```python
from build123d import *

# Parameters (mm, degrees)
SKETCH1_R                 = 1.143
BOSS_EXTRUDE1_DEPTH       = 3.9624
SKETCH2_W                 = 6.35
SKETCH2_H                 = 4.7752
BOSS_EXTRUDE2_DEPTH       = 7.2136
BOSS_EXTRUDE3_DEPTH       = 0.127
BOSS_EXTRUDE3_DEPTH_BACK  = 0.127
SKETCH3_R                 = 0.5588
BOSS_EXTRUDE4_DEPTH       = 0.127
BOSS_EXTRUDE4_DEPTH_BACK  = 0.127
SKETCH4_R                 = 0.5588
BOSS_EXTRUDE5_DEPTH       = 0.127
BOSS_EXTRUDE5_DEPTH_BACK  = 0.127
SKETCH5_R                 = 0.5588
BOSS_EXTRUDE6_DEPTH       = 0.127
BOSS_EXTRUDE6_DEPTH_BACK  = 0.127
SKETCH7_R                 = 0.5588
BOSS_EXTRUDE7_DEPTH       = 0.127
BOSS_EXTRUDE7_DEPTH_BACK  = 0.127
SKETCH6_R                 = 0.5588
BOSS_EXTRUDE8_DEPTH       = 0.0508
BOSS_EXTRUDE8_DEPTH_BACK  = 0.0508
BOSS_EXTRUDE11_DEPTH      = 0.0508
BOSS_EXTRUDE11_DEPTH_BACK = 0.0508
BOSS_EXTRUDE12_DEPTH      = 0.0508
BOSS_EXTRUDE12_DEPTH_BACK = 0.0508
BOSS_EXTRUDE13_DEPTH      = 0.0508
BOSS_EXTRUDE13_DEPTH_BACK = 0.0508
BOSS_EXTRUDE14_DEPTH      = 0.0508
BOSS_EXTRUDE14_DEPTH_BACK = 0.0508
BOSS_EXTRUDE15_DEPTH      = 0.0508
BOSS_EXTRUDE15_DEPTH_BACK = 0.0508
BOSS_EXTRUDE16_DEPTH      = 0.0508
BOSS_EXTRUDE16_DEPTH_BACK = 0.0508
BOSS_EXTRUDE17_DEPTH      = 0.0508
BOSS_EXTRUDE17_DEPTH_BACK = 0.0508
BOSS_EXTRUDE18_DEPTH      = 0.127
BOSS_EXTRUDE18_DEPTH_BACK = 0.127
SKETCH16_R                = 0.5588
BOSS_EXTRUDE19_DEPTH      = 0.127
BOSS_EXTRUDE19_DEPTH_BACK = 0.127
SKETCH18_R                = 0.5588
BOSS_EXTRUDE20_DEPTH      = 0.127
BOSS_EXTRUDE20_DEPTH_BACK = 0.127
SKETCH17_R                = 0.5588


with BuildPart() as part:
    # Sketch1 → Boss-Extrude1 (new body)
    with BuildSketch(Plane.XY):
        with BuildLine():
            Line((-5.5499, 2.3876), (5.5499, 2.3876))
            ThreePointArc((5.5499, 2.3876), (7.9375, 0), (5.5499, -2.3876))
            Line((5.5499, -2.3876), (-5.5499, -2.3876))
            ThreePointArc((-5.5499, -2.3876), (-7.9375, 0), (-5.5499, 2.3876))
        make_face()
        with Locations((-5.5499, 0)):
            Circle(SKETCH1_R, mode=Mode.SUBTRACT)
        with Locations((5.5499, 0)):
            Circle(SKETCH1_R, mode=Mode.SUBTRACT)
    extrude(amount=BOSS_EXTRUDE1_DEPTH)

    # Sketch2 → Boss-Extrude2 (add)
    with BuildSketch(Plane.XY.offset(3.9624)):
        Rectangle(SKETCH2_W, SKETCH2_H)
    extrude(amount=BOSS_EXTRUDE2_DEPTH)

    # Sketch3 → Boss-Extrude3 (add, two sides: drawn at the far end of the back side and taken through both)
    with BuildSketch(Plane(origin=(0, 0, 1.651), x_dir=(-1, 0, 0), z_dir=(0, 0, -1)).offset(-BOSS_EXTRUDE3_DEPTH_BACK)):
        with BuildLine():
            Line((-2.3114, 3.5941), (-2.3114, 2.3876))
            Line((-2.3114, 2.3876), (0, 2.3876))
            Line((0, 2.3876), (0, 3.5941))
            ThreePointArc((0, 3.5941), (-1.1557, 4.7498), (-2.3114, 3.5941))
        make_face()
        with Locations((-1.1557, 3.5941)):
            Circle(SKETCH3_R, mode=Mode.SUBTRACT)
    extrude(amount=BOSS_EXTRUDE3_DEPTH + BOSS_EXTRUDE3_DEPTH_BACK)

    # Sketch4 → Boss-Extrude4 (add, two sides: drawn at the far end of the back side and taken through both)
    with BuildSketch(Plane(origin=(0, 0, 2.921), x_dir=(-1, 0, 0), z_dir=(0, 0, -1)).offset(-BOSS_EXTRUDE4_DEPTH_BACK)):
        with BuildLine():
            Line((2.3114, 3.5941), (2.3114, 2.3876))
            Line((2.3114, 2.3876), (0, 2.3876))
            Line((0, 2.3876), (0, 3.5941))
            ThreePointArc((0, 3.5941), (1.1557, 4.7498), (2.3114, 3.5941))
        make_face()
        with Locations(Location((1.1557, 3.5941, 0), (0, 0, 180))):
            Circle(SKETCH4_R, mode=Mode.SUBTRACT)
    extrude(amount=BOSS_EXTRUDE4_DEPTH + BOSS_EXTRUDE4_DEPTH_BACK)

    # Sketch5 → Boss-Extrude5 (add, two sides: drawn at the far end of the back side and taken through both)
    with BuildSketch(Plane(origin=(0, 0, 4.191), x_dir=(-1, 0, 0), z_dir=(0, 0, -1)).offset(-BOSS_EXTRUDE5_DEPTH_BACK)):
        with BuildLine():
            Line((-2.3114, 3.5941), (-2.3114, 2.3876))
            Line((-2.3114, 2.3876), (0, 2.3876))
            Line((0, 2.3876), (0, 3.5941))
            ThreePointArc((0, 3.5941), (-1.1557, 4.7498), (-2.3114, 3.5941))
        make_face()
        with Locations((-1.1557, 3.5941)):
            Circle(SKETCH5_R, mode=Mode.SUBTRACT)
    extrude(amount=BOSS_EXTRUDE5_DEPTH + BOSS_EXTRUDE5_DEPTH_BACK)

    # Sketch7 → Boss-Extrude6 (add, two sides: drawn at the far end of the back side and taken through both)
    with BuildSketch(Plane(origin=(0, 0, 5.461), x_dir=(-1, 0, 0), z_dir=(0, 0, -1)).offset(-BOSS_EXTRUDE6_DEPTH_BACK)):
        with BuildLine():
            Line((2.3114, 2.3876), (2.3114, 3.5941))
            ThreePointArc((2.3114, 3.5941), (1.1557, 4.7498), (0, 3.5941))
            Line((0, 3.5941), (0, 2.3876))
            Line((0, 2.3876), (2.3114, 2.3876))
        make_face()
        with Locations(Location((1.1557, 3.5941, 0), (0, 0, 180))):
            Circle(SKETCH7_R, mode=Mode.SUBTRACT)
    extrude(amount=BOSS_EXTRUDE6_DEPTH + BOSS_EXTRUDE6_DEPTH_BACK)

    # Sketch6 → Boss-Extrude7 (add, two sides: drawn at the far end of the back side and taken through both)
    with BuildSketch(Plane(origin=(0, 0, 6.731), x_dir=(-1, 0, 0), z_dir=(0, 0, -1)).offset(-BOSS_EXTRUDE7_DEPTH_BACK)):
        with BuildLine():
            Line((-2.3114, 3.5941), (-2.3114, 2.3876))
            Line((-2.3114, 2.3876), (0, 2.3876))
            Line((0, 2.3876), (0, 3.5941))
            ThreePointArc((0, 3.5941), (-1.1557, 4.7498), (-2.3114, 3.5941))
        make_face()
        with Locations((-1.1557, 3.5941)):
            Circle(SKETCH6_R, mode=Mode.SUBTRACT)
    extrude(amount=BOSS_EXTRUDE7_DEPTH + BOSS_EXTRUDE7_DEPTH_BACK)

    # Sketch8 → Boss-Extrude8 (add, two sides: drawn at the far end of the back side and taken through both)
    with BuildSketch(Plane(origin=(0, 0, 1.651), x_dir=(-1, 0, 0), z_dir=(0, 0, -1)).offset(-BOSS_EXTRUDE8_DEPTH_BACK)):
        Polygon((2.228681211, -2.3876), (2.028101851, -2.3876), (0.796265448, -10.3124), (0.900870757, -10.3124), align=None)
        Polygon((-0.900870757, -10.3124), (-0.796265448, -10.3124), (-2.028101851, -2.3876), (-2.228681211, -2.3876), align=None)
    extrude(amount=BOSS_EXTRUDE8_DEPTH + BOSS_EXTRUDE8_DEPTH_BACK)

    # Sketch11 → Boss-Extrude11 (add, two sides: drawn at the far end of the back side and taken through both)
    with BuildSketch(Plane(origin=(0, 0, 4.191), x_dir=(-1, 0, 0), z_dir=(0, 0, -1)).offset(-BOSS_EXTRUDE11_DEPTH_BACK)):
        Polygon((2.228681211, -2.3876), (0.900870757, -10.3124), (0.796265448, -10.3124), (2.028101851, -2.3876), align=None)
        Polygon((-0.900870757, -10.3124), (-0.796265448, -10.3124), (-2.028101851, -2.3876), (-2.228681211, -2.3876), align=None)
    extrude(amount=BOSS_EXTRUDE11_DEPTH + BOSS_EXTRUDE11_DEPTH_BACK)

    # Sketch12 → Boss-Extrude12 (add, two sides: drawn at the far end of the back side and taken through both)
    with BuildSketch(Plane(origin=(0, 0, 6.731), x_dir=(-1, 0, 0), z_dir=(0, 0, -1)).offset(-BOSS_EXTRUDE12_DEPTH_BACK)):
        Polygon((2.228681211, -2.3876), (0.900870757, -10.3124), (0.796265448, -10.3124), (2.028101851, -2.3876), align=None)
        Polygon((-0.900870757, -10.3124), (-0.796265448, -10.3124), (-2.028101851, -2.3876), (-2.228681211, -2.3876), align=None)
    extrude(amount=BOSS_EXTRUDE12_DEPTH + BOSS_EXTRUDE12_DEPTH_BACK)

    # Sketch13 → Boss-Extrude13 (add, two sides: drawn at the far end of the back side and taken through both)
    with BuildSketch(Plane(origin=(0, 0, 2.921), x_dir=(-1, 0, 0), z_dir=(0, 0, -1)).offset(-BOSS_EXTRUDE13_DEPTH_BACK)):
        Polygon((0.900870757, -10.3124), (0.796265448, -10.3124), (2.028101851, -2.3876), (2.228681211, -2.3876), align=None)
        Polygon((-0.900870757, -10.3124), (-0.796265448, -10.3124), (-2.028101851, -2.3876), (-2.228681211, -2.3876), align=None)
    extrude(amount=BOSS_EXTRUDE13_DEPTH + BOSS_EXTRUDE13_DEPTH_BACK)

    # Sketch15 → Boss-Extrude14 (add, two sides: drawn at the far end of the back side and taken through both)
    with BuildSketch(Plane(origin=(0, 0, 5.461), x_dir=(-1, 0, 0), z_dir=(0, 0, -1)).offset(-BOSS_EXTRUDE14_DEPTH_BACK)):
        Polygon((-0.900870757, -10.3124), (-2.228681211, -2.3876), (-2.028101851, -2.3876), (-0.796265448, -10.3124), align=None)
        Polygon((0.796265448, -10.3124), (0.900870757, -10.3124), (2.228681211, -2.3876), (2.028101851, -2.3876), align=None)
    extrude(amount=BOSS_EXTRUDE14_DEPTH + BOSS_EXTRUDE14_DEPTH_BACK)

    # Sketch21 → Boss-Extrude15 (add, two sides: drawn at the far end of the back side and taken through both)
    with BuildSketch(Plane(origin=(0, 0, 10.541), x_dir=(-1, 0, 0), z_dir=(0, 0, -1)).offset(-BOSS_EXTRUDE15_DEPTH_BACK)):
        Polygon((-2.028101851, -2.3876), (-0.796265448, -10.3124), (-0.900870757, -10.3124), (-2.228681211, -2.3876), align=None)
        Polygon((0.796265448, -10.3124), (0.900870757, -10.3124), (2.228681211, -2.3876), (2.028101851, -2.3876), align=None)
    extrude(amount=BOSS_EXTRUDE15_DEPTH + BOSS_EXTRUDE15_DEPTH_BACK)

    # Sketch20 → Boss-Extrude16 (add, two sides: drawn at the far end of the back side and taken through both)
    with BuildSketch(Plane(origin=(0, 0, 9.271), x_dir=(-1, 0, 0), z_dir=(0, 0, -1)).offset(-BOSS_EXTRUDE16_DEPTH_BACK)):
        Polygon((2.228681211, -2.3876), (0.900870757, -10.3124), (0.796265448, -10.3124), (2.028101851, -2.3876), align=None)
        Polygon((-0.900870757, -10.3124), (-0.796265448, -10.3124), (-2.028101851, -2.3876), (-2.228681211, -2.3876), align=None)
    extrude(amount=BOSS_EXTRUDE16_DEPTH + BOSS_EXTRUDE16_DEPTH_BACK)

    # Sketch19 → Boss-Extrude17 (add, two sides: drawn at the far end of the back side and taken through both)
    with BuildSketch(Plane(origin=(0, 0, 8.001), x_dir=(-1, 0, 0), z_dir=(0, 0, -1)).offset(-BOSS_EXTRUDE17_DEPTH_BACK)):
        Polygon((-2.028101851, -2.3876), (-0.796265448, -10.3124), (-0.900870757, -10.3124), (-2.228681211, -2.3876), align=None)
        Polygon((0.796265448, -10.3124), (0.900870757, -10.3124), (2.228681211, -2.3876), (2.028101851, -2.3876), align=None)
    extrude(amount=BOSS_EXTRUDE17_DEPTH + BOSS_EXTRUDE17_DEPTH_BACK)

    # Sketch16 → Boss-Extrude18 (add, two sides: drawn at the far end of the back side and taken through both)
    with BuildSketch(Plane(origin=(0, 0, 8.001), x_dir=(-1, 0, 0), z_dir=(0, 0, -1)).offset(-BOSS_EXTRUDE18_DEPTH_BACK)):
        with BuildLine():
            Line((2.3114, 2.3876), (2.3114, 3.5941))
            ThreePointArc((2.3114, 3.5941), (1.1557, 4.7498), (0, 3.5941))
            Line((0, 3.5941), (0, 2.3876))
            Line((0, 2.3876), (2.3114, 2.3876))
        make_face()
        with Locations(Location((1.1557, 3.5941, 0), (0, 0, 180))):
            Circle(SKETCH16_R, mode=Mode.SUBTRACT)
    extrude(amount=BOSS_EXTRUDE18_DEPTH + BOSS_EXTRUDE18_DEPTH_BACK)

    # Sketch18 → Boss-Extrude19 (add, two sides: drawn at the far end of the back side and taken through both)
    with BuildSketch(Plane(origin=(0, 0, 10.541), x_dir=(-1, 0, 0), z_dir=(0, 0, -1)).offset(-BOSS_EXTRUDE19_DEPTH_BACK)):
        with BuildLine():
            Line((2.3114, 2.3876), (2.3114, 3.5941))
            ThreePointArc((2.3114, 3.5941), (1.1557, 4.7498), (0, 3.5941))
            Line((0, 3.5941), (0, 2.3876))
            Line((0, 2.3876), (2.3114, 2.3876))
        make_face()
        with Locations(Location((1.1557, 3.5941, 0), (0, 0, 180))):
            Circle(SKETCH18_R, mode=Mode.SUBTRACT)
    extrude(amount=BOSS_EXTRUDE19_DEPTH + BOSS_EXTRUDE19_DEPTH_BACK)

    # Sketch17 → Boss-Extrude20 (add, two sides: drawn at the far end of the back side and taken through both)
    with BuildSketch(Plane(origin=(0, 0, 9.271), x_dir=(-1, 0, 0), z_dir=(0, 0, -1)).offset(-BOSS_EXTRUDE20_DEPTH_BACK)):
        with BuildLine():
            Line((-2.3114, 3.5941), (-2.3114, 2.3876))
            Line((-2.3114, 2.3876), (0, 2.3876))
            Line((0, 2.3876), (0, 3.5941))
            ThreePointArc((0, 3.5941), (-1.1557, 4.7498), (-2.3114, 3.5941))
        make_face()
        with Locations((-1.1557, 3.5941)):
            Circle(SKETCH17_R, mode=Mode.SUBTRACT)
    extrude(amount=BOSS_EXTRUDE20_DEPTH + BOSS_EXTRUDE20_DEPTH_BACK)


solid = part.part
```
Work out the finished part from the listing and answer in its coordinate system (mm). A direction names the side the tool comes from. Round coordinates to 2 decimals unless told otherwise and drop trailing zeros. Loops run counter-clockwise (first coordinate to the right, second up) from the corner with the lowest first, then second, coordinate; pieces in that order, holes last.
(1) For faces 1 (the flat face through (4.5, -1, 3.962)), 2 (the flat face through (2, 3, 9.144)), determine the directions among +Z, -Z, +X, -X, +Y, -Y from which every point of the face is accessible in a straight line to the end or side of a thin tool.
Computed values:
face 1: +Z, +X, +Y, -Y
face 2: +X, -X, +Y
(2) Each of these flat-tipped pins is pushed along its axis until it touches: P1, Ø1.6, axis at x = 1.5, y = -6, coming from the -Z side; P2, Ø1.8, axis at x = 0.5, y = 3.5, coming from the -Z side; P3, Ø1.6, axis at x = 1.5, y = -5.5, coming from the +Z side. Where does it stop, or does it pass through?
Computed values:
P1: stops at z = 1.6
P2: stops at z = 1.52
P3: stops at z = 10.59
(3) Find the intervals of material crossed by L1, parallel to X at y = -1, z = 10.5 (3 decimals); L2, parallel to Y at x = 0.75, z = 7; L3, parallel to Z at x = -4.75, y = 2.25, in increasing order.
Computed values:
L1: x = -3.175 to 3.175
L2: y = -2.39 to 2.39
L3: z = 0 to 3.96
(4) The part is cut by section C-C, the plane x = 5. Give the vertices of the cut face in (y, z).
Computed values:
outline: (-2.39, 0) - (-1, 0) - (-1, 3.96) - (-2.39, 3.96) - close; (1, 0) - (2.39, 0) - (2.39, 3.96) - (1, 3.96) - close
(5) The part is cut by section B-B, the plane y = 2.75. Give the number of separate pieces and of enclosed holes in the cut face, and give its area (3 significant figures).
Computed values:
separate pieces: 8
enclosed holes: 0
area: 4.70 mm2
(6) The part is cut by section A-A, the plane y = 0. Give the vertices of the cut face in (x, z) (1 decimal), and give its area (3 significant figures).
Computed values:
outline: (-7.9, 0) - (-6.7, 0) - (-6.7, 4) - (-7.9, 4) - close; (-4.4, 0) - (4.4, 0) - (4.4, 4) - (3.2, 4) - (3.2, 11.2) - (-3.2, 11.2) - (-3.2, 4) - (-4.4, 4) - close; (6.7, 0) - (7.9, 0) - (7.9, 4) - (6.7, 4) - close
area: 90.6 mm2
(7) The mould has two halves that part along Y. Classify faces 3 (the cylindrical face through (-4.494, -0.438, 1.953)), 4 (the flat face through (3.175, 0, 8)): pulls with the +Y half, pulls with the -Y half, needs draft (parallel to the pull), parting line crosses it, or undercut.
Computed values:
face 3: undercut
face 4: needs draft
